Verification items for the finished model (mm, model axes). Face numbers are marked on the shaded views. A direction names the side the tool comes from. Round coordinates to 2 decimals unless told otherwise and drop trailing zeros. Write each loop counter-clockwise with the first axis right and the second up, starting at its lowest first coordinate (ties: lowest second). Pieces come first, ordered by that corner, then holes.
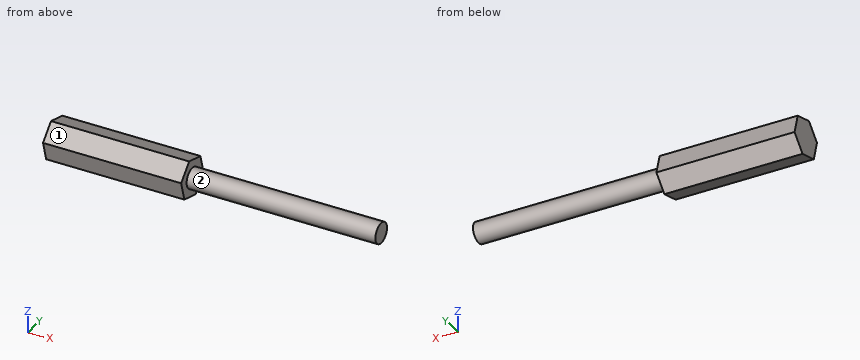
from build123d import *

# Parameters (mm, degrees)
F0_R     = 28.195536
F1_DEPTH = 355.6
F3_DEPTH = 190.5


with BuildPart() as f1:
    # F0 (on Right) → F1 (new body, symmetric)
    with BuildSketch(Plane.YZ):
        Circle(F0_R)
    extrude(amount=F1_DEPTH, both=True)

    # F2 (on face) → F3 (join, symmetric)
    with BuildSketch(Plane(origin=(-355.6, 0, 0), x_dir=(0, -1, 0), z_dir=(-1, 0, 0))):
        Polygon((54.718636, 13.456735), (15.705444, 54.116097), (-39.013193, 40.659361), (-54.718636, -13.456735), (-15.705444, -54.116097), (39.013193, -40.659361), align=None)
    extrude(amount=F3_DEPTH, both=True)


solid = f1.part
Q1. Sectioned sample at A-A (x = -297.5). Enter the section's corners in (y, z), plus the area to 3 significant figures.
Recorded:
outline: (-54.72, 13.46) - (-39.01, -40.66) - (15.71, -54.12) - (54.72, -13.46) - (39.01, 40.66) - (-15.71, 54.12) - close
area: 8,250 mm2
Q2. Material ranges on line 1 along X through (y, z) = (-26.5, 15); line 2 along Y through (x, z) = (287, -12); line 3 along Y through (x, z) = (-301, 19.5), recorded low to high.
Recorded:
line 1: x = -546.1 to -165.1
line 2: y = -25.51 to 25.51
line 3: y = -48.92 to 45.15
Q3. Sectioned sample at B-B (y = 0). Enter the section's corners in (x, z), plus the area to 3 significant figures.
Recorded:
outline: (-546.1, -50.25) - (-165.1, -50.25) - (-165.1, -28.2) - (355.6, -28.2) - (355.6, 28.2) - (-165.1, 28.2) - (-165.1, 50.25) - (-546.1, 50.25) - close
area: 67,700 mm2
Q4. Depth check by flat-ended pin: P1, Ø1.5, axis at x = -211, y = -15, coming from the -Z side; P2, Ø4, axis at x = -432, y = -21, coming from the -Z side; P3, Ø8, axis at x = -328, z = 40.5, coming from the +Y side. Enter the tip coordinate at first touch or a pass-through.
Recorded:
P1: stops at z = -46.75
P2: stops at z = -45.58
P3: stops at y = 40.22
Q5. Sectioned sample at C-C (z = 0). Enter the section's corners in (x, y), plus the area to 3 significant figures.
Recorded:
outline: (-546.1, -50.81) - (-165.1, -50.81) - (-165.1, -28.2) - (355.6, -28.2) - (355.6, 28.2) - (-165.1, 28.2) - (-165.1, 50.81) - (-546.1, 50.81) - close
area: 68,100 mm2
Q6. Tool access check on the marked faces 1 and 2. Record the directions out of +Z, -Z, +X, -X, +Y, -Y that give a thin tool (end or side, any length) a straight path to the whole face; none if there is none.
Recorded:
face 1: +Z, +X, -X, -Y
face 2: +X
Q7. Sectioned sample at D-D (x = -111.5). Enter the section's corners in (y, z), plus the area to 3 significant figures.
Recorded:
outline: circle Ø56.39 at (0, 0)
area: 2,500 mm2
